```python
from build123d import *

# Parameters (mm, degrees)
MODEL_R                 = 1.5
SALIENTE_EXTRUIR1_DEPTH = 3


with BuildPart() as part:
    # Model → Saliente-Extruir1 (new body)
    with BuildSketch(Plane.XY):
        with BuildLine():
            Line((-1396.348255289, 396.908179756), (-1470.105614602, 396.908179756))
            ThreePointArc((-1470.105614602, 396.908179756), (-1470.679639751, 396.793999055), (-1471.166274774, 396.468839928))
            Line((-1471.166274774, 396.468839928), (-1479.287595118, 388.347519585))
            ThreePointArc((-1479.287595118, 388.347519585), (-1479.612754245, 387.860884562), (-1479.726934946, 387.286859413))
            Line((-1479.726934946, 387.286859413), (-1479.726934946, 329.408179756))
            Line((-1479.726934946, 329.408179756), (-1470.731934946, 329.408179756))
            Line((-1470.731934946, 329.408179756), (-1470.731934946, 330.658179756))
            ThreePointArc((-1470.731934946, 330.658179756), (-1470.512265032, 331.188509842), (-1469.981934946, 331.408179756))
            Line((-1469.981934946, 331.408179756), (-1468.231934946, 331.408179756))
            ThreePointArc((-1468.231934946, 331.408179756), (-1467.70160486, 331.188509842), (-1467.481934946, 330.658179756))
            Line((-1467.481934946, 330.658179756), (-1467.481934946, 329.408179756))
            Line((-1467.481934946, 329.408179756), (-1463.856934946, 329.408179756))
            ThreePointArc((-1463.856934946, 329.408179756), (-1463.32660486, 329.188509842), (-1463.106934946, 328.658179756))
            Line((-1463.106934946, 328.658179756), (-1463.106934946, 327.158179756))
            ThreePointArc((-1463.106934946, 327.158179756), (-1463.32660486, 326.627849671), (-1463.856934946, 326.408179756))
            Line((-1463.856934946, 326.408179756), (-1467.481934946, 326.408179756))
            Line((-1467.481934946, 326.408179756), (-1467.481934946, 325.158179756))
            ThreePointArc((-1467.481934946, 325.158179756), (-1467.70160486, 324.627849671), (-1468.231934946, 324.408179756))
            Line((-1468.231934946, 324.408179756), (-1469.981934946, 324.408179756))
            ThreePointArc((-1469.981934946, 324.408179756), (-1470.512265032, 324.627849671), (-1470.731934946, 325.158179756))
            Line((-1470.731934946, 325.158179756), (-1470.731934946, 326.408179756))
            Line((-1470.731934946, 326.408179756), (-1479.726934946, 326.408179756))
            Line((-1479.726934946, 326.408179756), (-1479.726934946, 317.408179756))
            ThreePointArc((-1479.726934946, 317.408179756), (-1479.287595118, 316.347519585), (-1478.226934946, 315.908179756))
            Line((-1478.226934946, 315.908179756), (-1388.226934946, 315.908179756))
            ThreePointArc((-1388.226934946, 315.908179756), (-1387.166274774, 316.347519585), (-1386.726934946, 317.408179756))
            Line((-1386.726934946, 317.408179756), (-1386.726934946, 326.408179756))
            Line((-1386.726934946, 326.408179756), (-1395.721934946, 326.408179756))
            Line((-1395.721934946, 326.408179756), (-1395.721934946, 325.158179756))
            ThreePointArc((-1395.721934946, 325.158179756), (-1395.94160486, 324.627849671), (-1396.471934946, 324.408179756))
            Line((-1396.471934946, 324.408179756), (-1398.221934946, 324.408179756))
            ThreePointArc((-1398.221934946, 324.408179756), (-1398.752265032, 324.627849671), (-1398.971934946, 325.158179756))
            Line((-1398.971934946, 325.158179756), (-1398.971934946, 326.408179756))
            Line((-1398.971934946, 326.408179756), (-1402.596934946, 326.408179756))
            ThreePointArc((-1402.596934946, 326.408179756), (-1403.127265032, 326.627849671), (-1403.346934946, 327.158179756))
            Line((-1403.346934946, 327.158179756), (-1403.346934946, 328.658179756))
            ThreePointArc((-1403.346934946, 328.658179756), (-1403.127265032, 329.188509842), (-1402.596934946, 329.408179756))
            Line((-1402.596934946, 329.408179756), (-1398.971934946, 329.408179756))
            Line((-1398.971934946, 329.408179756), (-1398.971934946, 330.658179756))
            ThreePointArc((-1398.971934946, 330.658179756), (-1398.752265032, 331.188509842), (-1398.221934946, 331.408179756))
            Line((-1398.221934946, 331.408179756), (-1396.471934946, 331.408179756))
            ThreePointArc((-1396.471934946, 331.408179756), (-1395.94160486, 331.188509842), (-1395.721934946, 330.658179756))
            Line((-1395.721934946, 330.658179756), (-1395.721934946, 329.408179756))
            Line((-1395.721934946, 329.408179756), (-1386.726934946, 329.408179756))
            Line((-1386.726934946, 329.408179756), (-1386.726934946, 387.286859413))
            ThreePointArc((-1386.726934946, 387.286859413), (-1386.841115647, 387.860884562), (-1387.166274774, 388.347519585))
            Line((-1387.166274774, 388.347519585), (-1395.287595118, 396.468839928))
            ThreePointArc((-1395.287595118, 396.468839928), (-1395.774230141, 396.793999055), (-1396.348255289, 396.908179756))
        make_face()
        with Locations((-1433.226934946, 392.408179756)):
            Circle(MODEL_R, mode=Mode.SUBTRACT)
        with Locations((-1451.226934946, 392.408179756)):
            Circle(MODEL_R, mode=Mode.SUBTRACT)
        with Locations((-1442.226934946, 392.408179756)):
            Circle(MODEL_R, mode=Mode.SUBTRACT)
        with Locations((-1442.226934946, 383.408179756)):
            Circle(MODEL_R, mode=Mode.SUBTRACT)
        with Locations((-1433.226934946, 383.408179756)):
            Circle(MODEL_R, mode=Mode.SUBTRACT)
        with Locations((-1451.226934946, 383.408179756)):
            Circle(MODEL_R, mode=Mode.SUBTRACT)
        with Locations((-1424.226934946, 392.408179756)):
            Circle(MODEL_R, mode=Mode.SUBTRACT)
        with Locations((-1415.226934946, 392.408179756)):
            Circle(MODEL_R, mode=Mode.SUBTRACT)
        with Locations((-1424.226934946, 383.408179756)):
            Circle(MODEL_R, mode=Mode.SUBTRACT)
        with Locations((-1457.226934946, 327.908179756)):
            Circle(MODEL_R, mode=Mode.SUBTRACT)
        with Locations((-1409.226934946, 327.908179756)):
            Circle(MODEL_R, mode=Mode.SUBTRACT)
        with Locations((-1415.226934946, 383.408179756)):
            Circle(MODEL_R, mode=Mode.SUBTRACT)
    extrude(amount=SALIENTE_EXTRUIR1_DEPTH)


solid = part.part
```
Work out the finished part from the listing and answer in its coordinate system (mm). A direction names the side the tool comes from. Coordinates: 2 decimals unless noted, no trailing zeros. Use CSV: the item, a comma, the result in double quotes. Start each with the question number.
(1) Consider line 1 (X direction, y = 330, z = 1.5); line 2 (Y direction, x = -1423, z = 0.15); line 3 (Y direction, x = -1401, z = 2.3). Determine where each line is inside the solid, lowest interval first.
(2) For a pull along Y with two mould halves and no side action, classify faces 4 (the face through (-1458.42, 327, 1.48)), 5 (the face through (-1434, 315.908, 1)), 6 (the face through (-1433, 396.908, 1)), 7 (the face through (-1386.727, 322, 1)) as +Y half, -Y half, draft (parallel to the pull), parting line (faces both ways), or undercut.
(3) Find section A-A, the plane z = 2.2. State how many separate pieces and enclosed holes the cut face has, then the cut area to 3 significant figures.
(4) For faces 1 (the face through (-1391, 329.408, 1)), 2 (the face through (-1466, 329.408, 1)), 3 (the face through (-1479.727, 322, 1)), determine the directions among +Z, -Z, +X, -X, +Y, -Y from which every point of the face is accessible in a straight line to the end or side of a thin tool.
(5) Given pin 1 Ø2.5 at (x, y) = (-1415.23, 383.41) entering from -Z, flat-ended and moving along its own axis, determine where the tip first touches the part or whether it passes through.
Recorded:
1,line 1,"x = -1479.73 to -1470.73, -1467.48 to -1398.97, -1395.72 to -1386.73"
1,line 2,"y = 315.91 to 382.55, 384.27 to 391.55, 393.27 to 396.91"
1,line 3,"y = 315.91 to 326.41, 329.41 to 396.91"
2,face 4,"undercut"
2,face 5,"-Y half"
2,face 6,"+Y half"
2,face 7,"draft"
3,separate pieces,"1"
3,enclosed holes,"12"
3,area,"7,240 mm^2"
4,face 1,"+Z, -Z, +X"
4,face 2,"+Z, -Z, -X"
4,face 3,"+Z, -Z, -X, +Y, -Y"
5,pin 1,"passes through"
